For this review, use the dimensioned drawing (mm, ordinates from the lowest corner) and the shaded views. Coordinates: 2 decimals unless noted, no trailing zeros. Loops run counter-clockwise (first coordinate to the right, second up) from the corner with the lowest first, then second, coordinate; pieces in that order, holes last. Notation, with made-up numbers: (76.5, -6.75) - (115.5, -6.75) arc R18 ccw to (115.5, 21.25) - close; hole circle Ø5 at (73, -38.5). An arc over 180 degrees is marked (long way). Use one line per item in the form item = value. Start each with the question number.
(1) Clearance check with a flat-ended pin moving along its axis: pin 1 Ø8 at (x, y) = (447, 23.5) entering from +Z. State where the tip first meets the part, or that it passes through.
(2) Add section A-A (y = 40). State the section outline as (x, z) points.
(3) For L1, parallel to Y at x = 440.5, z = 4.75; L2, parallel to Y at x = 82, z = 28.75; L3, parallel to X at y = 32, z = 23.25, list the stretches that pass through material, from the lowest coordinate up.
(4) Add section C-C (z = 8). State the section outline as (x, y) points, plus the area to 3 significant figures.
(5) Add section B-B (x = 430). State the section outline as (y, z) points.
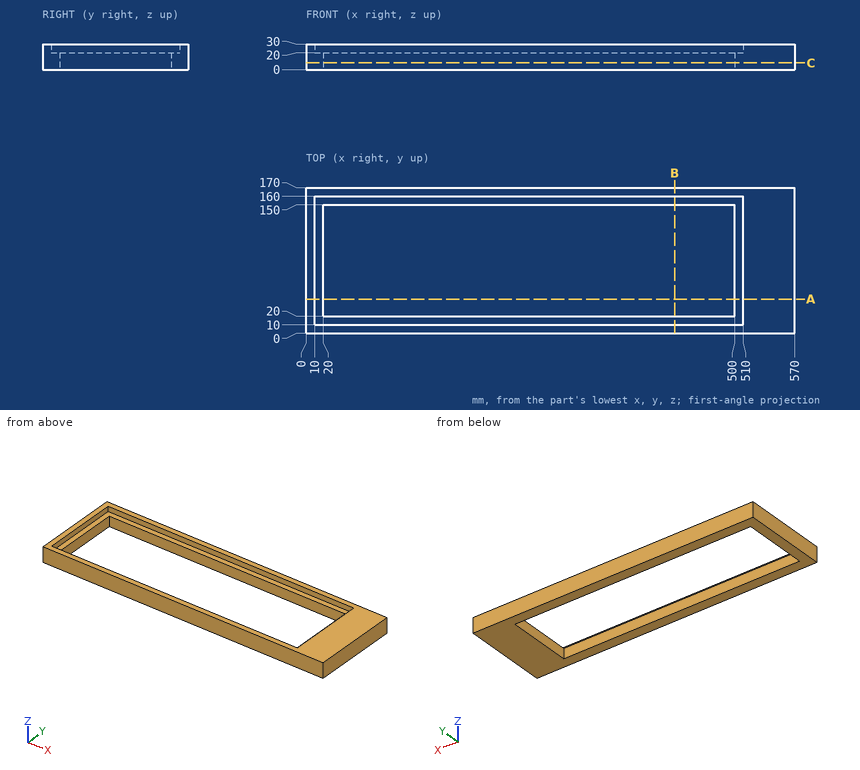
Computed values:
q1.pin_1 = 20
q2.outline = (0, 0) - (20, 0) - (20, 20) - (10, 20) - (10, 30) - (0, 30) - close; (500, 0) - (570, 0) - (570, 30) - (510, 30) - (510, 20) - (500, 20) - close
q3.L1 = 0 to 20, 150 to 170
q3.L2 = 0 to 10, 160 to 170
q3.L3 = 0 to 10, 510 to 570
q4.outline = (0, 0) - (570, 0) - (570, 170) - (0, 170) - close; hole (20, 20) - (500, 20) - (500, 150) - (20, 150) - close
q4.area = 34,500 mm^2
q5.outline = (0, 0) - (20, 0) - (20, 20) - (10, 20) - (10, 30) - (0, 30) - close; (150, 0) - (170, 0) - (170, 30) - (160, 30) - (160, 20) - (150, 20) - close
